from build123d import *

# Parameters (mm, degrees)
SKETCH1_W           = 45
SKETCH1_H           = 80
BOSS_EXTRUDE1_DEPTH = 3.175
SKETCH2_W           = 15
SKETCH2_H           = 6.35
CUT_EXTRUDE1_DEPTH  = 92.842695001
SKETCH3_R           = 1.5
SKETCH3_W           = 30
SKETCH3_H           = 60.825
CUT_EXTRUDE2_DEPTH  = 92.842695001
FILLET1_R           = 10
FILLET2_R           = 2


with BuildPart() as part:
    # Sketch1 → Boss-Extrude1 (new body)
    with BuildSketch(Plane.XY):
        with Locations((-22.5, -40)):
            Rectangle(SKETCH1_W, SKETCH1_H)
    extrude(amount=BOSS_EXTRUDE1_DEPTH)

    # Sketch2 → Cut-Extrude1 (cut, through all)
    with BuildSketch(Plane.XY.offset(3.175)):
        with Locations((0, -10)):
            Rectangle(SKETCH2_W, SKETCH2_H)
    extrude(amount=-CUT_EXTRUDE1_DEPTH, mode=Mode.SUBTRACT)

    # Sketch3 → Cut-Extrude2 (cut, through all)
    with BuildSketch(Plane.XY.offset(3.175)):
        with Locations((-37.5, -74)):
            Circle(SKETCH3_R)
        with Locations((-15, -49.5875)):
            Rectangle(SKETCH3_W, SKETCH3_H)
    extrude(amount=-CUT_EXTRUDE2_DEPTH, mode=Mode.SUBTRACT)

    # Fillet1
    fillet1_edges = [part.edges().sort_by_distance(p)[0] for p in [
        (-30, -19.175, 1.5875),
        (-45, 0, 1.5875),
    ]]
    fillet(fillet1_edges, radius=FILLET1_R)

    # Fillet2
    fillet2_edges = [part.edges().sort_by_distance(p)[0] for p in [
        (0, -13.175, 1.5875),
        (0, -6.825, 1.5875),
        (0, -19.175, 1.5875),
        (0, 0, 1.5875),
    ]]
    fillet(fillet2_edges, radius=FILLET2_R)


solid = part.part
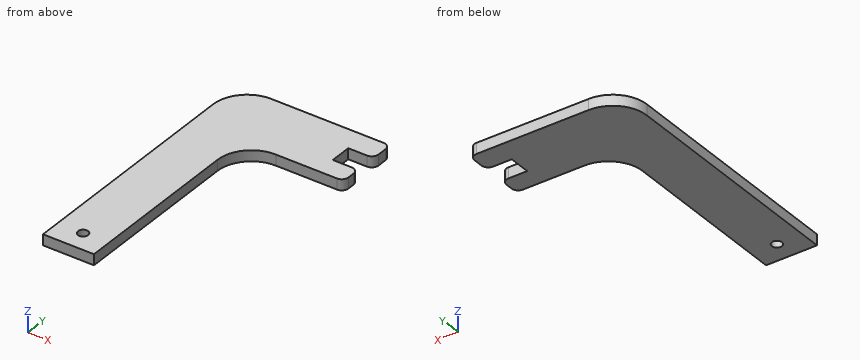
CAD build for the part. Positions are in the model's coordinates, mm. Round coordinates to 2 decimals unless told otherwise and drop trailing zeros. Order: outer loops, then holes, each group sorted by start corner. A loop starts at its lowest first (then second) coordinate and runs counter-clockwise, first axis right, second up. Notation, with made-up numbers: (27.25, -1) -> (50.25, -1) arc R17 cw to (50.25, 18) -> close; hole circle Ø5 at (28.5, -1.5). An arc over 180 degrees is marked (long way). Write item = value, one per line. Start each with the question number.
(1) Cut at A-A, the plane z = 1.3. List the corners of the cut face in (x, y) (3 decimals), then the cut area to 3 significant figures.
(2) Cut at B-B, the plane y = -74. List the corners of the cut face in (x, z) (3 decimals), then the cut area to 3 significant figures.
(3) Cut at C-C, the plane x = -38. List the corners of the cut face in (y, z) (3 decimals), then the cut area to 3 significant figures.
(4) Cut at D-D, the plane x = -13. List the corners of the cut face in (y, z) (3 decimals).
(5) Pin check, flat tips, straight feed: P1, Ø2.5, axis at x = -37.5, y = -74, coming from the -Z side; P2, Ø1.6, axis at x = -7.5, z = 2, coming from the -Y side (3 decimals); P3, Ø1.6, axis at y = -47.5, z = 2, coming from the +X side; P4, Ø1, axis at y = -10.5, z = 1, coming from the +X side. Stop position of each tip, or through.
(6) Probe line 1 (X direction, y = -74, z = 1.5); line 2 (Y direction, x = -6, z = 2.15) (3 decimals); line 3 (Y direction, x = -35.5, z = 1.7). List the from-to ranges inside material, lowest first. Write a range as [from, to].
Model answer:
q1.outline = (-45, -80) -> (-30, -80) -> (-30, -29.175) arc R10 cw to (-20, -19.175) -> (-2, -19.175) arc R2 ccw to (0, -17.175) -> (0, -15.175) arc R2 ccw to (-2, -13.175) -> (-7.5, -13.175) -> (-7.5, -6.825) -> (-2, -6.825) arc R2 ccw to (0, -4.825) -> (0, -2) arc R2 ccw to (-2, 0) -> (-35, 0) arc R10 ccw to (-45, -10) -> close; hole circle Ø3 at (-37.5, -74)
q1.area = 1,720 mm2
q2.outline = (-45, 0) -> (-39, 0) -> (-39, 3.175) -> (-45, 3.175) -> close; (-36, 0) -> (-30, 0) -> (-30, 3.175) -> (-36, 3.175) -> close
q2.area = 38.1 mm2
q3.outline = (-80, 0) -> (-75.414, 0) -> (-75.414, 3.175) -> (-80, 3.175) -> close; (-72.586, 0) -> (-0.461, 0) -> (-0.461, 3.175) -> (-72.586, 3.175) -> close
q3.area = 244 mm2
q4.outline = (-19.175, 0) -> (0, 0) -> (0, 3.175) -> (-19.175, 3.175) -> close
q5.P1 = through
q5.P2 = -19.175
q5.P3 = -30
q5.P4 = -7.5
q6.line_1 = [-45, -39], [-36, -30]
q6.line_2 = [-19.175, -13.175], [-6.825, 0]
q6.line_3 = [-80, -0.01]
